from build123d import *

# Parameters (mm, degrees)
F1_R     = 11
F1_R_2   = 8.2
F1_R_3   = 6.2
F2_DEPTH = 22
F3_DEPTH = 18
F4_DEPTH = 6


with BuildPart() as f2:
    # F1 (on Right) → F2 (new body, through all)
    with BuildSketch(Plane.YZ):
        Circle(F1_R)
        Circle(F1_R_2, mode=Mode.SUBTRACT)
        Circle(F1_R_2)
        Circle(F1_R_3, mode=Mode.SUBTRACT)
        Circle(F1_R_3)
    extrude(amount=-F2_DEPTH)

    # F1 (on Right) → F3 (join, through all)
    with BuildSketch(Plane.YZ):
        Circle(F1_R_3)
    extrude(amount=F3_DEPTH)

    # F1 (on Right) → F4 (join, through all)
    with BuildSketch(Plane.YZ):
        Circle(F1_R_2)
        Circle(F1_R_3, mode=Mode.SUBTRACT)
    extrude(amount=F4_DEPTH)


with BuildPart() as f2_1:
    # F5: moved
    add(f2.part.moved(Location((22, 0, 0))))


solid = f2_1.part
Geometry check sheet. Reference: the model listing, model coordinates, mm. A direction names the side the tool comes from. Give positions to 0.01 mm unless a question says otherwise; leave off trailing zeros. Loops run counter-clockwise (first coordinate to the right, second up) from the corner with the lowest first, then second, coordinate; pieces in that order, holes last. Notation, with made-up numbers: (-15.5, 73.5) -> (29.5, 73.5) arc R30 ccw to (29.5, 104.5) -> close; hole circle Ø5 at (-8.5, 54.25). An arc over 180 degrees is marked (long way). Answer in a Markdown table with one row per item. Add a question column.
1) Set-up check for faces 1 (the face through (0, 0, 0)), 2 (the face through (24.96, -1.07, 8.13)): record each of +Z, -Z, +X, -X, +Y, -Y from which the full face is reachable in a straight line by a thin tool's end or side.
2) Gauge pin test, flat ends, axial feed: P1, Ø3, axis at x = 22.5, z = 6, coming from the -Y side; P2, Ø10, axis at y = -5.5, z = 8.5, coming from the +X side; P3, Ø1.5, axis at x = 31, y = -2.5, coming from the -Z side; P4, Ø10, axis at x = 30.5, y = -5, coming from the -Z side. Record the tip position at first contact, or that the pin passes through.
3) Material ranges on probe 1 along X at (y, z) = (7.25, -2.75); probe 2 along X at (y, z) = (-7.25, -6.25); probe 3 along Y at (x, z) = (25, 0.25), recorded low to high. Write a range as from..to.
4) Cross-section at A-A on y = 0. Record the boundary of the cut face in (x, z), and give its area (3 significant figures).
5) Cross-section at D-D on y = 7.5. Record the boundary of the cut face in (x, z).
6) Cross-section at C-C on x = 38. Record the boundary of the cut face in (y, z), and give its area (3 significant figures).
Outcome:
| question | item | result |
|---|---|---|
| 1 | face 1 | +Z, -Z, -X, +Y, -Y |
| 1 | face 2 | +X |
| 2 | P1 | stops at y = -10 |
| 2 | P2 | stops at x = 40 |
| 2 | P3 | stops at z = -5.95 |
| 2 | P4 | stops at z = -8.17 |
| 3 | probe 1 | x = 0..28 |
| 3 | probe 2 | x = 0..22 |
| 3 | probe 3 | y = -8.2..8.2 |
| 4 | outline | (0, -11) -> (22, -11) -> (22, -8.2) -> (28, -8.2) -> (28, -6.2) -> (40, -6.2) -> (40, 6.2) -> (28, 6.2) -> (28, 8.2) -> (22, 8.2) -> (22, 11) -> (0, 11) -> close |
| 4 | area | 731 mm^2 |
| 5 | outline | (0, -8.05) -> (22, -8.05) -> (22, -3.32) -> (28, -3.32) -> (28, 3.32) -> (22, 3.32) -> (22, 8.05) -> (0, 8.05) -> close |
| 6 | outline | circle Ø12.4 at (0, 0) |
| 6 | area | 121 mm^2 |
